Here's how the part is built. I have some questions about the finished solid (model axes, mm). Face numbers are marked on the shaded views. A direction names the side the tool comes from. Give positions to 0.01 mm unless a question says otherwise; leave off trailing zeros. Loops run counter-clockwise (first coordinate to the right, second up) from the corner with the lowest first, then second, coordinate; pieces in that order, holes last. Notation, with made-up numbers: (52, 37.5) -> (60, 37.5) arc R29 cw to (60, 76.5) -> close; hole circle Ø2 at (28.5, 47). An arc over 180 degrees is marked (long way). Answer in a Markdown table with one row per item. Add a question column.
Item 1: If we section it at C-C (y = -17): Write out the boundary of the cut face in (x, z).
Item 2: Which directions (+Z, -Z, +X, -X, +Y, -Y) give clear straight access to the entire face, cutting with the end or side of a thin tool? Please do the marked faces 4, 5 and 6.
Item 3: If we section it at D-D (y = 5.5): Write out the boundary of the cut face in (x, z).
Item 4: For P1, Ø17.5, axis at x = 31.5, y = -0.5, coming from the +Z side; P2, Ø1.8, axis at x = -20, z = 11, coming from the -Y side; P3, Ø2, axis at x = -6.5, z = 4, coming from the +Y side; P4, Ø6.5, axis at x = -19, z = 4, coming from the +Y side, each with a flat end and sliding along its axis, tell me the tip position at first contact or that it passes through.
Item 5: We'd pull the mould along Y, two halves only. Please class the marked faces 1, 2 and 3: released by +Y, released by -Y, zero draft, split by the parting line, or undercut.
Item 6: If we section it at A-A (x = -20): Write out the boundary of the cut face in (y, z), then the cut area to 3 significant figures.
Item 7: If we section it at B-B (z = 7): Write out the boundary of the cut face in (x, y).
Item 8: If I drill on line 1 (Y direction, x = 27, z = 12.75); line 2 (Y direction, x = -19.5, z = 10.75); line 3 (X direction, y = -8, z = 0.75), over which ranges is the centre line in solid material (lowest first)?
```python
from build123d import *

# Parameters (mm, degrees)
SKETCH1_R           = 4.25
BOSS_EXTRUDE1_DEPTH = 15
SKETCH2_R           = 11.05
CUT_EXTRUDE1_DEPTH  = 10
SKETCH3_R           = 6
CUT_EXTRUDE2_DEPTH  = 10
CUT_EXTRUDE5_DEPTH  = 15


with BuildPart() as part:
    # Sketch1 → Boss-Extrude1 (new body)
    with BuildSketch(Plane.XY):
        with BuildLine():
            Line((-16.865782324, -15.62917697), (13.134217676, -15.62917697))
            ThreePointArc((13.134217676, -15.62917697), (48.706833622, -3.016216146), (13.054918576, 9.37082303))
            Line((13.054918576, 9.37082303), (-16.945081424, 9.37082303))
            ThreePointArc((-16.945081424, 9.37082303), (-40.196781878, -3.203056293), (-16.865782324, -15.62917697))
        make_face()
        with Locations((-25.196857337, -3.155477073)):
            Circle(SKETCH1_R, mode=Mode.SUBTRACT)
    extrude(amount=BOSS_EXTRUDE1_DEPTH)

    # Sketch2 → Cut-Extrude1 (cut)
    with BuildSketch(Plane.XY.offset(15)):
        with Locations((28.706934234, -3.079655107)):
            Circle(SKETCH2_R)
    extrude(amount=-CUT_EXTRUDE1_DEPTH, mode=Mode.SUBTRACT)

    # Sketch3 → Cut-Extrude2 (cut)
    with BuildSketch(Plane.XY.offset(5)):
        with Locations((28.706934234, -3.079655107)):
            Circle(SKETCH3_R)
    extrude(amount=-CUT_EXTRUDE2_DEPTH, mode=Mode.SUBTRACT)

    # Sketch5 → Cut-Extrude5 (cut)
    with BuildSketch(Plane.XY.offset(15)):
        with BuildLine():
            Line((-16.186458693, -0.155477073), (-22.186458693, -0.155477073))
            ThreePointArc((-22.186458693, -0.155477073), (-29.446857337, -3.155477073), (-22.186458693, -6.155477073))
            Line((-22.186458693, -6.155477073), (-16.186458693, -6.155477073))
            Line((-16.186458693, -6.155477073), (-16.186458693, -0.155477073))
        make_face()
    extrude(amount=-CUT_EXTRUDE5_DEPTH, mode=Mode.SUBTRACT)


solid = part.part
```
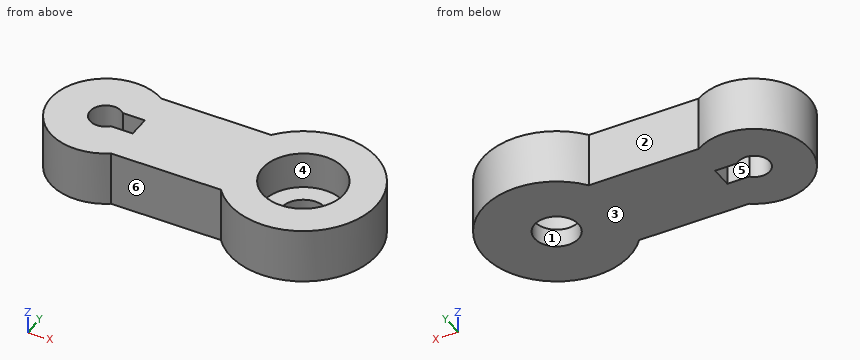
Recorded:
| question | item | result |
|---|---|---|
| 1 | outline | (-30.97, 0) -> (-19.42, 0) -> (-19.42, 15) -> (-30.97, 15) -> close; (14.35, 0) -> (43.07, 0) -> (43.07, 15) -> (14.35, 15) -> close |
| 2 | face 4 | +Z |
| 2 | face 5 | +Z, -Z |
| 2 | face 6 | +Z, -Z, -Y |
| 3 | outline | (-37.45, 0) -> (46.77, 0) -> (46.77, 15) -> (35.67, 15) -> (35.67, 5) -> (21.74, 5) -> (21.74, 15) -> (-37.45, 15) -> close |
| 4 | P1 | stops at z = 15 |
| 4 | P2 | stops at y = -17.53 |
| 4 | P3 | stops at y = 9.37 |
| 4 | P4 | stops at y = 11.55 |
| 5 | face 1 | undercut |
| 5 | face 2 | released by +Y |
| 5 | face 3 | zero draft |
| 6 | outline | (-17.23, 0) -> (-6.16, 0) -> (-6.16, 15) -> (-17.23, 15) -> close; (-0.16, 0) -> (10.92, 0) -> (10.92, 15) -> (-0.16, 15) -> close |
| 6 | area | 332 mm^2 |
| 7 | outline | (-16.95, 9.37) arc R15 ccw (long way) to (-16.87, -15.63) -> (13.13, -15.63) arc R20 ccw (long way) to (13.05, 9.37) -> close; hole (-22.19, -6.16) -> (-16.19, -6.16) -> (-16.19, -0.16) -> (-22.19, -0.16) arc R4.25 ccw (long way) to start; hole circle Ø22.1 at (28.71, -3.08) |
| 8 | line 1 | y = -23.01 to -14, 7.84 to 16.85 |
| 8 | line 2 | y = -17.03 to -6.16, -0.16 to 10.72 |
| 8 | line 3 | x = -39.39 to 25.27, 32.14 to 48.09 |
